from build123d import *

# Parameters (mm, degrees)
F0_R      = 50.1
F0_R_2    = 4.5
F1_DEPTH  = 3
F1_FACE_R = 50.1
F2_DEPTH  = 1
F3_R      = 4.5
F4_DEPTH  = 25


with BuildPart() as f1:
    # F0 (on Front) → F1 (new body)
    with BuildSketch(Plane.XZ):
        Circle(F0_R)
        Circle(F0_R_2, mode=Mode.SUBTRACT)
        Circle(F0_R_2)
    extrude(amount=F1_DEPTH)

    # F0 (on Front) + F1_face (on face) → F2 (join)
    with BuildSketch(Plane.XZ):
        Circle(F0_R)
        Circle(F0_R_2, mode=Mode.SUBTRACT)
    with BuildSketch(Plane.XZ.offset(3)):
        Circle(F1_FACE_R)
    extrude(amount=-F2_DEPTH)

    # F3 (on face) → F4 (cut)
    with BuildSketch(Plane.XZ.offset(3)):
        Circle(F3_R)
    extrude(amount=-F4_DEPTH, mode=Mode.SUBTRACT)


solid = f1.part
Work out the finished part from the listing and answer in its coordinate system (mm). Round coordinates to 2 decimals unless told otherwise and drop trailing zeros. Write each loop counter-clockwise with the first axis right and the second up, starting at its lowest first coordinate (ties: lowest second). Pieces come first, ordered by that corner, then holes.
1) Straight lines are drawn through the part: line 1 (Z direction, x = 0, y = 0.7); line 2 (Z direction, x = 1, y = -0.85); line 3 (X direction, y = 0.1, z = -10). For each, find the intervals that lie inside material, in ascending order.
2) Given pin 1 Ø1 at (y, z) = (0.5, -7) entering from -X; pin 2 Ø5.5 at (x, z) = (0, 0) entering from +Y; pin 3 Ø1.5 at (y, z) = (0, 23) entering from -X; pin 4 Ø1.5 at (y, z) = (-2, 27) entering from +X, each flat-ended and moving along its own axis, determine where each tip first touches the part or whether it passes through.
3) A cutting plane is placed at D-D (x = 38.5). Give the vertices of the cut face in (y, z), plus the area to 3 significant figures.
4) A cutting plane is placed at C-C (y = -1.35). Give the vertices of the cut face in (x, z), plus the area to 3 significant figures.
5) A cutting plane is placed at B-B (x = 0). Give the vertices of the cut face in (y, z).
6) A cutting plane is placed at A-A (z = 0). Give the vertices of the cut face in (x, y).
Completed:
1. line 1: z = -50.1 to -4.5, 4.5 to 50.1
1. line 2: z = -50.09 to -4.39, 4.39 to 50.09
1. line 3: x = -49.09 to 49.09
2. pin 1: stops at x = -49.68
2. pin 2: passes through
2. pin 3: stops at x = -44.89
2. pin 4: stops at x = 42.67
3. outline: (-3, -32.06) - (1, -32.06) - (1, 32.06) - (-3, 32.06) - close
3. area: 256 mm2
4. outline: circle Ø100.2 at (0, 0); hole circle Ø9 at (0, 0)
4. area: 7,820 mm2
5. outline: (-3, -50.1) - (1, -50.1) - (1, -4.5) - (-3, -4.5) - close; (-3, 4.5) - (1, 4.5) - (1, 50.1) - (-3, 50.1) - close
6. outline: (-50.1, -3) - (-4.5, -3) - (-4.5, 1) - (-50.1, 1) - close; (4.5, -3) - (50.1, -3) - (50.1, 1) - (4.5, 1) - close
